Design review of the part shown in the three views and the two pictorial views. Dimensions are in mm from the part's minimum x, y and z. Give positions to 0.01 mm unless a question says otherwise; leave off trailing zeros. Loops run counter-clockwise (first coordinate to the right, second up) from the corner with the lowest first, then second, coordinate; pieces in that order, holes last.
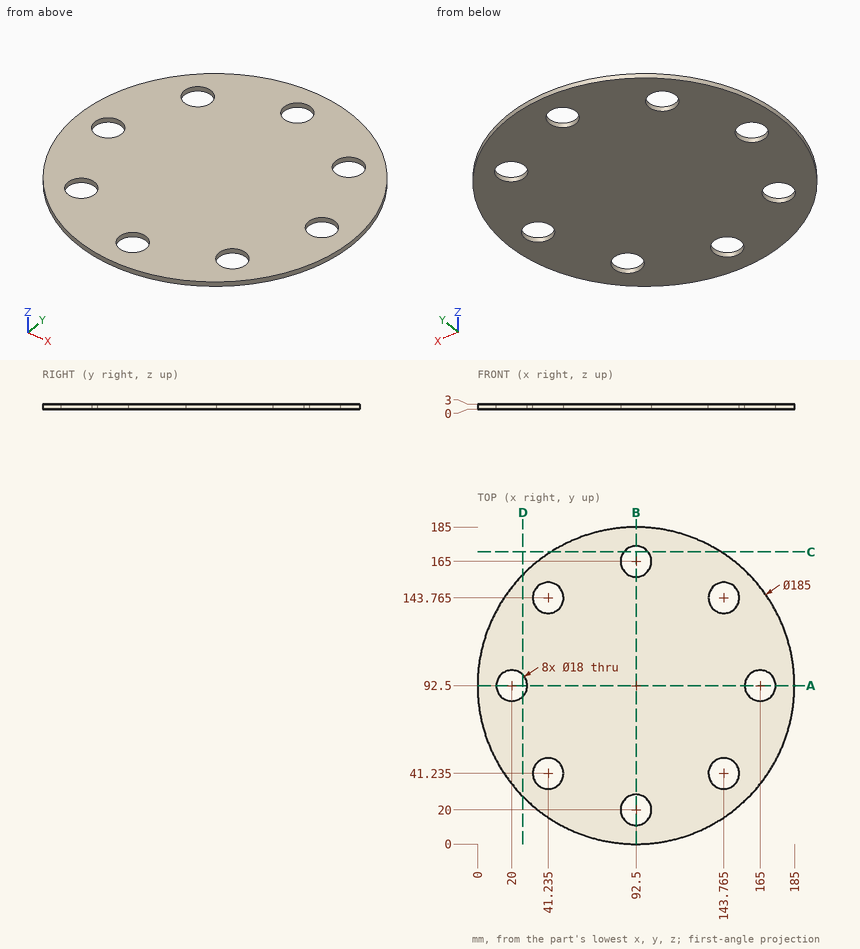
Q1. Consider section C-C on y = 170.5. Give the boundary of the cut face in (x, z).
Answers:
outline: (42.78, 0) - (85.38, 0) - (85.38, 3) - (42.78, 3) - close; (99.62, 0) - (142.22, 0) - (142.22, 3) - (99.62, 3) - close
Q2. Consider section A-A on y = 92.5. Give the boundary of the cut face in (x, z), plus the area to 3 significant figures.
Answers:
outline: (0, 0) - (11, 0) - (11, 3) - (0, 3) - close; (29, 0) - (156, 0) - (156, 3) - (29, 3) - close; (174, 0) - (185, 0) - (185, 3) - (174, 3) - close
area: 447 mm2
Q3. For probe 1 along Y at (x, z) = (92.5, 1.2); probe 2 along X at (y, z) = (43.5, 1.9) (1 decimal); probe 3 along X at (y, z) = (93.5, 1.2) (1 decimal), list the stretches that pass through material, from the lowest coordinate up.
Answers:
probe 1: y = 0 to 11, 29 to 156, 174 to 185
probe 2: x = 14 to 32.5, 49.9 to 135.1, 152.5 to 171
probe 3: x = 0 to 11.1, 28.9 to 156.1, 173.9 to 185
Q4. For pin 1 Ø16 at (x, y) = (41.23, 41.23) entering from +Z (1 decimal), flat-tipped, find the tip position at first contact; note if it passes through.
Answers:
pin 1: passes through
Q5. Consider section D-D on x = 26.5. Give the boundary of the cut face in (y, z) (1 decimal).
Answers:
outline: (27.7, 0) - (86.3, 0) - (86.3, 3) - (27.7, 3) - close; (98.7, 0) - (157.3, 0) - (157.3, 3) - (98.7, 3) - close
